The model under review builds one solid part; all positions refer to its coordinate system, in mm. Face numbers are marked on the shaded views. A direction names the side the tool comes from. Give positions to 0.01 mm unless a question says otherwise; leave off trailing zeros. Write each loop counter-clockwise with the first axis right and the second up, starting at its lowest first coordinate (ties: lowest second). Pieces come first, ordered by that corner, then holes. Notation, with made-up numbers: (75.5, 26) - (109.5, 26) arc R18 cw to (109.5, 49) - close; hole circle Ø2 at (62.5, 38). An arc over 180 degrees is marked (long way). One line per question, with ' | ' between items. Start each with the question number.
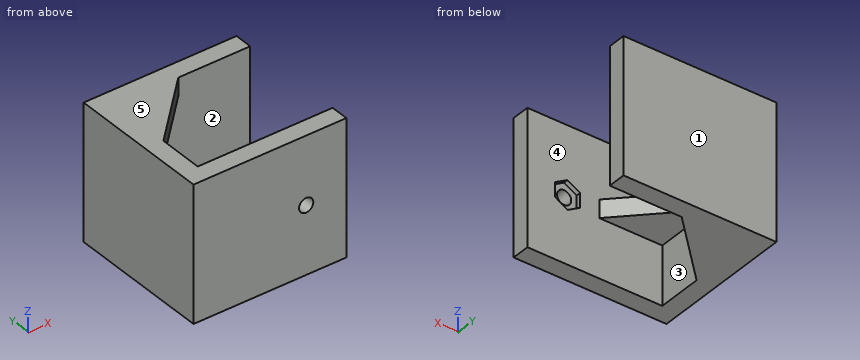
```python
from build123d import *

# Parameters (mm, degrees)
SKETCH1_W                = 68
SKETCH1_H                = 60
BOSS_EXTRUDE1_DEPTH      = 8
SKETCH4_W                = 8
SKETCH4_H                = 60
BOSS_EXTRUDE2_DEPTH      = 56
SKETCH5_R                = 3.175
CUT_EXTRUDE1_DEPTH       = 8
SKETCH6_W                = 60
SKETCH6_H                = 8
BOSS_EXTRUDE3_DEPTH      = 60
BOSS_EXTRUDE4_DEPTH      = 8
BOSS_EXTRUDE5_DEPTH      = 4
BOSS_EXTRUDE5_DEPTH_BACK = 4
CUT_EXTRUDE2_DEPTH       = 2


with BuildPart() as part:
    # Sketch1 → Boss-Extrude1 (new body)
    with BuildSketch(Plane(origin=(0, 0, 0), x_dir=(1, 0, 0), z_dir=(0, 1, 0))):
        with Locations((34, 30)):
            Rectangle(SKETCH1_W, SKETCH1_H)
    extrude(amount=BOSS_EXTRUDE1_DEPTH)

    # Sketch4 → Boss-Extrude2 (add)
    with BuildSketch(Plane(origin=(0, 8, 0), x_dir=(1, 0, 0), z_dir=(0, 1, 0))):
        with Locations((4, 30)):
            Rectangle(SKETCH4_W, SKETCH4_H)
    extrude(amount=BOSS_EXTRUDE2_DEPTH)

    # Sketch5 → Cut-Extrude1 (cut)
    with BuildSketch(Plane(origin=(0, 8, 0), x_dir=(1, 0, 0), z_dir=(0, 1, 0))):
        with Locations(Location((50.125, 30, 0), (0, 0, 270))):
            Circle(SKETCH5_R)
    extrude(amount=-CUT_EXTRUDE1_DEPTH, mode=Mode.SUBTRACT)

    # Sketch6 → Boss-Extrude3 (add)
    with BuildSketch(Plane(origin=(8, 0, 0), x_dir=(0, 0, -1), z_dir=(1, 0, 0))):
        with Locations((30, 60)):
            Rectangle(SKETCH6_W, SKETCH6_H)
    extrude(amount=BOSS_EXTRUDE3_DEPTH)

    # Sketch7 → Boss-Extrude4 (add)
    with BuildSketch(Plane.XY):
        Polygon((8, 56), (8, 28), (36, 56), align=None)
    boss_extrude4 = extrude(amount=-BOSS_EXTRUDE4_DEPTH)

    # Mirror1: Boss-Extrude4 across plane
    add(boss_extrude4.mirror(Plane.XY.offset(-30)))

    # Sketch8 → Boss-Extrude5 (add, two sides: drawn at the far end of the back side and taken through both)
    with BuildSketch(Plane.XY.offset(-30).offset(-BOSS_EXTRUDE5_DEPTH_BACK)):
        Polygon((8, 36), (8, 8), (36, 8), align=None)
    extrude(amount=BOSS_EXTRUDE5_DEPTH + BOSS_EXTRUDE5_DEPTH_BACK)

    # Sketch9 → Cut-Extrude2 (cut)
    with BuildSketch(Plane(origin=(0, 8, 0), x_dir=(1, 0, 0), z_dir=(0, 1, 0))):
        Polygon((50.125, 36.415804866), (44.56875, 33.207902433), (44.56875, 26.792097567), (50.125, 23.584195134), (55.68125, 26.792097567), (55.68125, 33.207902433), align=None)
    extrude(amount=-CUT_EXTRUDE2_DEPTH, mode=Mode.SUBTRACT)


solid = part.part
```
Item 1: Take a section at A-A (x = 14.5). Give the boundary of the cut face in (y, z), plus the area to 3 significant figures.
Item 2: Machinability: for the marked faces 1 and 2, which of the approach directions +Z, -Z, +X, -X, +Y, -Y give a long, thin tool a straight path to every point of the face, cutting with its end or side? Answer none if there is none.
Item 3: The part is to be moulded in two halves that separate along Z. For the marked faces 3, 4 and 5, say which applies: +Z half, -Z half, draft (parallel to the pull), parting line (faces both ways), or undercut.
Item 4: Clearance check with flat-ended pins moving along their axes: P1, Ø7.5, axis at x = 50.125, z = -30, coming from the -Y side; P2, Ø6, axis at y = 43.5, z = -11.5, coming from the +X side; P3, Ø24, axis at y = 21.5, z = -42.5, coming from the +X side. State where each tip first meets the part, or that it passes through.
Item 5: Take a section at D-D (x = 21.5). Give the boundary of the cut face in (y, z), plus the area to 3 significant figures.
Item 6: Take a section at C-C (y = 52). Give the boundary of the cut face in (x, z), plus the area to 3 significant figures.
Item 7: For probe 1 along Z at (x, y) = (19, 46.5); probe 2 along Y at (x, z) = (45, -6); probe 3 along X at (y, z) = (3.6, -30), list the stretches that pass through material, from the lowest coordinate up.
Item 8: Take a section at B-B (z = -30). Give the boundary of the cut face in (x, y).
Check sheet entries:
1) outline: (0, -60) - (8, -60) - (8, -34) - (29.5, -34) - (29.5, -26) - (8, -26) - (8, 0) - (0, 0) - close; (34.5, -60) - (64, -60) - (64, 0) - (34.5, 0) - (34.5, -8) - (56, -8) - (56, -52) - (34.5, -52) - close | area: 1,480 mm^2
2) face 1: +Z, -Z, +X, -X, +Y | face 2: +X
3) face 3: undercut | face 4: draft | face 5: +Z half
4) P1: stops at y = 0 | P2: stops at x = 8 | P3: stops at x = 30.97
5) outline: (0, -60) - (8, -60) - (8, -34) - (22.5, -34) - (22.5, -26) - (8, -26) - (8, 0) - (0, 0) - close; (41.5, -60) - (64, -60) - (64, 0) - (41.5, 0) - (41.5, -8) - (56, -8) - (56, -52) - (41.5, -52) - close | area: 1,310 mm^2
6) outline: (0, -60) - (32, -60) - (32, -52) - (8, -52) - (8, -8) - (32, -8) - (32, 0) - (0, 0) - close | area: 864 mm^2
7) probe 1: z = -60 to -52, -8 to 0 | probe 2: y = 0 to 8, 56 to 64 | probe 3: x = 0 to 46.95, 53.3 to 68
8) outline: (0, 0) - (46.95, 0) - (46.95, 6) - (44.57, 6) - (44.57, 8) - (36, 8) - (8, 36) - (8, 56) - (68, 56) - (68, 64) - (0, 64) - close; (53.3, 0) - (68, 0) - (68, 8) - (55.68, 8) - (55.68, 6) - (53.3, 6) - close
